```python
from build123d import *

# Parameters (mm, degrees)
MODEL_W                 = 5
MODEL_H                 = 3
SALIENTE_EXTRUIR1_DEPTH = 3


with BuildPart() as part:
    # Model → Saliente-Extruir1 (new body)
    with BuildSketch(Plane.XY):
        with BuildLine():
            ThreePointArc((41.267867754, 50.3668743), (41.840038745, 49.712625685), (42.516862734, 49.167345775))
            ThreePointArc((42.516862734, 49.167345775), (46.658942321, 47.821013343), (50.890017113, 48.854183425))
            ThreePointArc((50.890017113, 48.854183425), (51.682739903, 49.412356399), (52.352838083, 50.113023882))
            ThreePointArc((52.352838083, 50.113023882), (55.298688256, 53.204742994), (58.776644321, 55.682762754))
            ThreePointArc((58.776644321, 55.682762754), (60.384709339, 56.272809284), (62.097562925, 56.285482302))
            ThreePointArc((62.097562925, 56.285482302), (66.436098934, 54.702702392), (69.908221839, 51.657632693))
            ThreePointArc((69.908221839, 51.657632693), (70.701503033, 50.2031837), (70.975974725, 48.569359286))
            Line((70.975974725, 48.569359286), (70.975974725, -12.270034891))
            ThreePointArc((70.975974725, -12.270034891), (68.051211593, -19.336931187), (60.987770072, -22.270027934))
            Line((60.987770072, -22.270027934), (14.985714259, -22.315810799))
            ThreePointArc((14.985714259, -22.315810799), (7.908350506, -19.39032634), (4.975973655, -12.315815543))
            Line((4.975973655, -12.315815543), (4.975973655, -2.813238517))
            Line((4.975973655, -2.813238517), (4.975973655, 40.425288245))
            Line((4.975973655, 40.425288245), (4.975973655, 49.884528276))
            ThreePointArc((4.975973655, 49.884528276), (8.113744062, 54.521049823), (13.601344724, 53.412368555))
            ThreePointArc((13.601344724, 53.412368555), (13.707091478, 53.309379729), (13.815832279, 53.209557326))
            ThreePointArc((13.815832279, 53.209557326), (17.640590842, 50.871877459), (22.042476183, 50.025159874))
            ThreePointArc((22.042476183, 50.025159874), (23.098925942, 50.126451448), (24.110198526, 50.448435664))
            ThreePointArc((24.110198526, 50.448435664), (28.729757377, 52.257521246), (33.482882411, 53.679110861))
            ThreePointArc((33.482882411, 53.679110861), (34.313026149, 53.81737559), (35.154600394, 53.814451111))
            ThreePointArc((35.154600394, 53.814451111), (38.583837662, 52.751366), (41.267867754, 50.3668743))
        make_face()
        with Locations((45.675973655, -16.835371011)):
            Rectangle(MODEL_W, MODEL_H, mode=Mode.SUBTRACT)
        with Locations((35.675973655, -16.835371011)):
            Rectangle(MODEL_W, MODEL_H, mode=Mode.SUBTRACT)
        with BuildLine():
            ThreePointArc((61.544611159, 47.747091698), (59.825660646, 48.823765634), (57.918666613, 48.13283048))
            ThreePointArc((57.918666613, 48.13283048), (57.495803013, 37.456958674), (64.907336248, 29.761360741))
            ThreePointArc((64.907336248, 29.761360741), (62.061503492, 32.95773428), (62.730808451, 37.184742531))
            ThreePointArc((62.730808451, 37.184742531), (63.597745225, 38.946667832), (63.936191604, 40.880941387))
            ThreePointArc((63.936191604, 40.880941387), (63.639107759, 44.627049101), (61.544611159, 47.747091698))
        make_face(mode=Mode.SUBTRACT)
        with BuildLine():
            ThreePointArc((37.783690328, 37.119649339), (40.764172897, 41.613475795), (40.490547933, 46.998908176))
            ThreePointArc((40.490547933, 46.998908176), (38.645359064, 48.710978233), (36.129518354, 48.791298643))
            ThreePointArc((36.129518354, 48.791298643), (34.308280563, 42.580138607), (37.783690328, 37.119649339))
        make_face(mode=Mode.SUBTRACT)
        with BuildLine():
            ThreePointArc((8.359011818, 41.762359599), (11.200768363, 39.871762064), (14.466790556, 40.863244963))
            ThreePointArc((14.466790556, 40.863244963), (14.466640554, 44.89370885), (12.048482223, 48.118169962))
            ThreePointArc((12.048482223, 48.118169962), (10.408906396, 48.767789115), (8.824071113, 47.99415415))
            ThreePointArc((8.824071113, 47.99415415), (7.978922821, 44.923974684), (8.359011818, 41.762359599))
        make_face(mode=Mode.SUBTRACT)
    extrude(amount=SALIENTE_EXTRUIR1_DEPTH)


solid = part.part
```
The listing builds one solid part. Answer for the finished solid, in the listing's coordinates (mm). A direction names the side the tool comes from. Coordinates: 2 decimals unless noted, no trailing zeros. Loops run counter-clockwise (first coordinate to the right, second up) from the corner with the lowest first, then second, coordinate; pieces in that order, holes last. Notation, with made-up numbers: (58.5, -32.5) - (86.5, -32.5) arc R23 ccw to (86.5, -5.5) - close; hole circle Ø8 at (-5.5, 88). An arc over 180 degrees is marked (long way). Write item = value, one per line.
1) Section D-D (x = 30) is taken. Determine the outline of the cut face in (y, z).
Responses:
outline = (-22.3, 0) - (52.68, 0) - (52.68, 3) - (-22.3, 3) - close
2) Section A-A (x = 39) is taken. Determine the outline of the cut face in (y, z), plus the area to 3 significant figures.
Responses:
outline = (-22.29, 0) - (38.29, 0) - (38.29, 3) - (-22.29, 3) - close; (48.54, 0) - (52.5, 0) - (52.5, 3) - (48.54, 3) - close
area = 194 mm^2
3) Find the intervals of material crossed by line 1 along X through (y, z) = (51, 2.7); line 2 along X through (y, z) = (32, 0.2); line 3 along X through (y, z) = (37.5, 1.65), in increasing order.
Responses:
line_1 = 5.11 to 17.32, 25.4 to 40.76, 53.09 to 70.35
line_2 = 4.98 to 61.31, 62.45 to 70.98
line_3 = 4.98 to 37.25, 38.23 to 57.48, 62.93 to 70.98
4) Section B-B (z = 1.4) is taken. Count the separate pieces of the cut face and the enclosed holes in it, plus the area to 3 significant figures.
Responses:
separate_pieces = 1
enclosed_holes = 5
area = 4,650 mm^2
5) Determine the mould class of faces 3 (the face through (36, -15.335, 1)), 4 (the face through (38, 18, 0)), 5 (the face through (63.656, 44.577, 1.479)), 6 (the face through (66.38, 54.736, 1.479)) for opening direction X: pulls with the +X half, pulls with the -X half, needs draft (parallel to the pull), parting line crosses it, or undercut.
Responses:
face_3 = undercut
face_4 = needs draft
face_5 = undercut
face_6 = pulls with the +X half
6) Each of these flat-tipped pins is pushed along its axis until it touches: P1, Ø0.9, axis at x = 36, z = 1, coming from the -Y side; P2, Ø0.9, axis at x = 35, z = 2, coming from the +Y side; P3, Ø0.9, axis at y = -16, z = 1.5, coming from the -X side. Where does it stop, or does it pass through?
Responses:
P1 = -22.3
P2 = 53.83
P3 = 5.51
7) Section C-C (x = 20) is taken. Determine the outline of the cut face in (y, z).
Responses:
outline = (-22.31, 0) - (50.21, 0) - (50.21, 3) - (-22.31, 3) - close
8) Which of the six approach directions +Z, -Z, +X, -X, +Y, -Y give full straight-line access (tool end or side, diameter ignored) to faces 1 (the face through (4.976, 18, 1)), 2 (the face through (40.744, 41.54, 1.479))?
Responses:
face_1 = +Z, -Z, -X, +Y, -Y
face_2 = +Z, -Z
